Autodesk Fusion 360 part; units mm, degrees
sketch "Esquisse7" plane through (0, 0, 10) normal (0, 0, 1) x (-1, 0, 0)
  circle A0 centre (-12, 0) radius 7.6
  circle A1 centre (12, 0) radius 7.6
  line L0 (-19.9, -8.9) -> (19.9, -8.9)
  line L1 (19.9, -8.9) -> (19.9, 8.9)
  line L2 (19.9, 8.9) -> (-19.9, 8.9)
  line L3 (-19.9, 8.9) -> (-19.9, -8.9)
  line L4 (0, 0) -> (-2.53, 5.0152)
sketch "Esquisse3" plane through (0, 0, 10) normal (0, 0, 1) x (-1, 0, 0)
  line L0 (21.15, -10.65) -> (-21.15, -10.65)
  line L1 (-21.15, -10.65) -> (-21.15, 10.65)
  line L2 (-21.15, 10.65) -> (21.15, 10.65)
  line L3 (21.15, 10.65) -> (21.15, -10.65)
  line L4 (21.15, -10.65) -> (-21.15, 10.65) construction
  line L5 (-21.15, -10.65) -> (21.15, 10.65) construction
  line L6 (22.5, -15) -> (-22.5, -15)
  line L7 (-22.5, -15) -> (-22.5, 15)
  line L8 (-22.5, 15) -> (22.5, 15)
  line L9 (22.5, 15) -> (22.5, -15)
  line L10 (22.5, -15) -> (-22.5, 15) construction
  line L11 (-22.5, -15) -> (22.5, 15) construction
  dimension "d76" = 42.3
  dimension "d77" = 21.3
  dimension "d78" = 45
  dimension "d79" = 30
extrude "Extrusion1" add sketch "Esquisse3" against normal blind 11
extrude "Extrusion2" add sketch "Esquisse3" along normal blind 1.5 contours L0 L1 L2 L3 | L6 L7 L8 L9
sketch "Esquisse4" plane through (0, -15, 0) normal (0, -1, 0) x (1, 0, 0)
  line L0 (-22.5, 11.5) -> (-22.5, -1)
  line L1 (-22.5, -1) -> (22.5, -1)
  line L2 (22.5, -1) -> (22.5, 11.5)
  line L3 (22.5, 11.5) -> (-22.5, 11.5)
  line L4 (0, 0) -> (0, 3.5)
  dimension "d84" = 3.5
hole "Perçage1" at (0, -15, 3.5) direction (0, 1, 0) diameter 3.3 depth 8 tip angle 180 counterbore diameter 5.8 counterbore depth 3
sketch "Esquisse5" plane through (0, 15, 0) normal (0, 1, 0) x (-1, 0, 0)
  line L0 (-22.5, 11.5) -> (-22.5, -1)
  line L1 (-22.5, -1) -> (22.5, -1)
  line L2 (22.5, -1) -> (22.5, 11.5)
  line L3 (22.5, 11.5) -> (-22.5, 11.5)
  line L4 (0, 0) -> (0, 3.5)
  dimension "d100" = 3.5
hole "Perçage2" at (0, 15, 3.5) direction (0, -1, 0) diameter 3.3 depth 8 tip angle 180 counterbore diameter 5.8 counterbore depth 3
hole "Perçage3" at (0, 0, 11.5) direction (0, 0, -1) diameter 8 depth 1.5 tip angle 180
sketch "Esquisse6" plane through (0, 0, -1) normal (0, 0, -1) x (1, 0, 0)
  line L0 (-21.15, 10.65) -> (21.15, 10.65)
  line L1 (21.15, 10.65) -> (21.15, -10.65)
  line L2 (21.15, -10.65) -> (-21.15, -10.65)
  line L3 (-21.15, -10.65) -> (-21.15, 10.65)
  line L4 (22.5, 15) -> (-22.5, 15)
  line L5 (-22.5, 15) -> (-22.5, -15)
  line L6 (-22.5, -15) -> (22.5, -15)
  line L7 (22.5, -15) -> (22.5, 15)
  line L8 (-22.5, 15) -> (-12.5, 15)
  circle A0 centre (-12.5, 15) radius 3.5
  line L9 (22.5, -15) -> (12.5, -15)
  circle A1 centre (12.5, -15) radius 3.5
  dimension "d119" = 7
  dimension "d120" = 10
  dimension "d121" = 7
extrude "Extrusion3" add sketch "Esquisse6" along normal blind 1 contours L4 L8 A0 | L6 L9 A1 picked at (-14.8203, 14.8261) picked at (10.334, -14.1499)
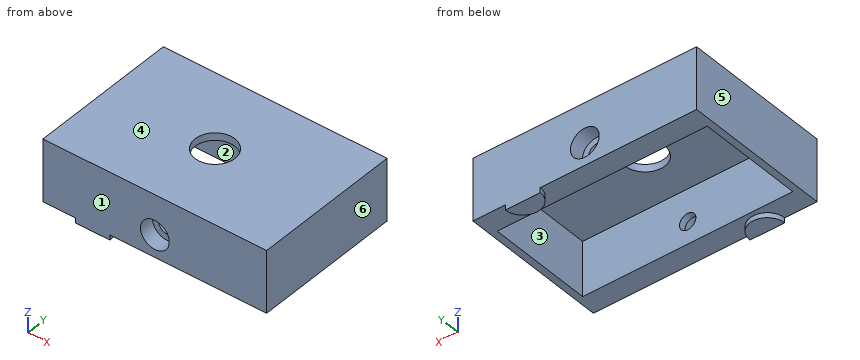
The listing builds one solid part. Answer for the finished solid, in the listing's coordinates (mm). Face numbers are marked on the shaded views. A direction names the side the tool comes from. Give positions to 0.01 mm unless a question says otherwise; leave off trailing zeros. Loops run counter-clockwise (first coordinate to the right, second up) from the corner with the lowest first, then second, coordinate; pieces in that order, holes last. Notation, with made-up numbers: M 50,24 L 56,24 A35 ccw 56,61 Z; hole C -34,-36.75 d10. An arc over 180 degrees is marked long. One line per item, written item: value.
Q1. A cutting plane is placed at A-A on z = 3.5. Determine the outline of the cut face in (x, y).
Working result:
outline: M -22.5,-15 L -2.9,-15 L -2.9,-12 L -1.65,-12 L -1.65,-10.65 L -21.15,-10.65 L -21.15,10.65 L -1.65,10.65 L -1.65,12 L -2.9,12 L -2.9,15 L -22.5,15 Z; M 1.65,-12 L 2.9,-12 L 2.9,-15 L 22.5,-15 L 22.5,15 L 2.9,15 L 2.9,12 L 1.65,12 L 1.65,10.65 L 21.15,10.65 L 21.15,-10.65 L 1.65,-10.65 Z
Q2. For the marked faces 1 and 2, determine the directions among +Z, -Z, +X, -X, +Y, -Y from which every point of the face is accessible in a straight line to the end or side of a thin tool.
Working result:
face 1: +Z, -Z, +X, -X, -Y
face 2: -Z
Q3. Determine the mould class of the marked faces 3, 4, 5 and 6 for opening direction X: +X half, -X half, draft (parallel to the pull), parting line (faces both ways), or undercut.
Working result:
face 3: undercut
face 4: draft
face 5: -X half
face 6: +X half
Q4. A cutting plane is placed at C-C on z = 9.25. Determine the outline of the cut face in (x, y), then the cut area to 3 significant figures.
Working result:
outline: M -22.5,-15 L 22.5,-15 L 22.5,15 L -22.5,15 Z; hole M -21.15,-10.65 L 21.15,-10.65 L 21.15,10.65 L -21.15,10.65 Z
area: 449 mm^2
Q5. Find the intervals of material crossed by line 1 (Y direction, x = -5.5, z = 6.25); line 2 (X direction, y = 13.95, z = 3.5); line 3 (X direction, y = 2.25, z = 4.25), in increasing order. Write a range as from..to.
Working result:
line 1: y = -15..-10.65, 10.65..15
line 2: x = -22.5..-2.9, 2.9..22.5
line 3: x = -22.5..-21.15, 21.15..22.5
Q6. Flat-ended cylindrical pins translate along their axes: P1, Ø1, axis at x = 1.5, z = 5, coming from the -Y side; P2, Ø2, axis at x = 14, y = 2, coming from the -Z side. Find the tip coordinate at first contact, or state that the pin passes through.
Working result:
P1: stops at y = -12
P2: stops at z = 10
Q7. A cutting plane is placed at D-D on x = -1. Determine the outline of the cut face in (y, z).
Working result:
outline: M -15,-1 L -10.65,-1 L -10.65,2.19 L -12,2.19 L -12,0.78 L -15,0.78 Z; M -15,6.22 L -12,6.22 L -12,4.81 L -10.65,4.81 L -10.65,10 L -3.87,10 L -3.87,11.5 L -15,11.5 Z; M 3.87,10 L 10.65,10 L 10.65,4.81 L 12,4.81 L 12,6.22 L 15,6.22 L 15,11.5 L 3.87,11.5 Z; M 10.65,-1 L 15,-1 L 15,0.78 L 12,0.78 L 12,2.19 L 10.65,2.19 Z
Q8. A cutting plane is placed at B-B on y = 0. Determine the outline of the cut face in (x, z).
Working result:
outline: M -22.5,-1 L -21.15,-1 L -21.15,10 L -4,10 L -4,11.5 L -22.5,11.5 Z; M 4,10 L 21.15,10 L 21.15,-1 L 22.5,-1 L 22.5,11.5 L 4,11.5 Z
